Build history of the part. All positions in model axes, mm. Face numbers are marked on the shaded views. A direction names the side the tool comes from. Give positions to 0.01 mm unless a question says otherwise; leave off trailing zeros. Order: outer loops, then holes, each group sorted by start corner. A loop starts at its lowest first (then second) coordinate and runs counter-clockwise, first axis right, second up. Notation, with made-up numbers: (63, 68.5) - (71, 68.5) arc R30 cw to (71, 104.5) - close; hole circle Ø1 at (49, 87). An arc over 180 degrees is marked (long way). Use a Markdown table: item, result. Add a question column.
(1) Slice it at D-D (y = 1). Write the cut outline in (x, z), then the cut area to 3 significant figures.
(2) Flat gauge pins, fed straight in: pin 1 (5 mm diameter, centred on x = -2.5, z = -12.5, fed in from +Y); pin 2 (1.5 mm diameter, centred on y = 2.5, z = -15, fed in from +X); pin 3 (4.5 mm diameter, centred on x = 11, y = 2.5, fed in from -Z); pin 4 (1 mm diameter, centred on y = -1.5, z = 15.5, fed in from -X). Where does each tip first touch, or does it go through?
(3) Slice it at B-B (z = 12.5). Write the cut outline in (x, y).
(4) Mould opens along X. For the marked faces 1, 2, 3 and 4 say: +X half, -X half, draft (parallel to the pull), parting line (faces both ways), or undercut.
(5) Slice it at A-A (x = -2.5). Write the cut outline in (y, z), then the cut area to 3 significant figures.
(6) Slice it at C-C (y = -1.5). Write the cut outline in (x, z).
(7) Which spindle directions (+Z, -Z, +X, -X, +Y, -Y) get a long thin tool onto all of the face, cutting with end or side? Do the marked faces 5, 6, 7, 8 and 9. Say none if no direction does.
(8) Wall check: line 1 (Z direction, x = -2.5, y = 1.55); line 2 (Z direction, x = 11.25, y = 4); line 3 (X direction, y = -1.5, z = 16.5). Give the ranges that are in metal, low to high.
from build123d import *

# Parameters (mm, degrees)
EXTRUDE_1_DEPTH              = 10
SKETCH_2_W                   = 16
SKETCH_2_H                   = 6.92820323
EXTRUDE_2_DEPTH              = 10
SKETCH_3_W                   = 10
SKETCH_3_H                   = 6.92820323
CUT_EXTRUDE_1_DEPTH          = 1.5
CUT_EXTRUDE_2_DEPTH          = 1.92820323
EXTRUDE_3_DEPTH              = 10
SKETCH_6_W                   = 14.5
SKETCH_6_H                   = 5
EXTRUDE_4_DEPTH              = 10
HOLE_WIZARD_3_0_3_1_D        = 3
HOLE_WIZARD_3_0_3_1_DEPTH    = 10
HOLE_WIZARD_M5_1_D           = 5.5
HOLE_WIZARD_M5_1_DEPTH       = 9.237604307
HOLE_WIZARD_M5_1_CSINK_D     = 11.2
HOLE_WIZARD_M5_1_CSINK_ANGLE = 90
HOLE_WIZARD_3_0_3_2_D        = 3
HOLE_WIZARD_3_0_3_2_DEPTH    = 30
CHAMFER_1_SIZE               = 2


with BuildPart() as part:
    # 草图1 → 凸台-拉伸1 (new body)
    with BuildSketch(Plane.XY):
        Polygon((10, 5), (-10, 5), (-10, -1.92820323), (6, -1.92820323), (10, -4.237604307), (14, -1.92820323), (14, 2.690598923), align=None)
    extrude(amount=-EXTRUDE_1_DEPTH)

    # 草图2 → 凸台-拉伸2 (add)
    with BuildSketch(Plane.XY):
        with Locations((-2, 1.535898385)):
            Rectangle(SKETCH_2_W, SKETCH_2_H)
    extrude(amount=EXTRUDE_2_DEPTH)

    # 草图3 → 切除-拉伸1 (cut)
    with BuildSketch(Plane(origin=(6, 0, 0), x_dir=(0, 0, -1), z_dir=(1, 0, 0))):
        with Locations((-5, 1.535898385)):
            Rectangle(SKETCH_3_W, SKETCH_3_H)
    extrude(amount=-CUT_EXTRUDE_1_DEPTH, mode=Mode.SUBTRACT)

    # 草图4 → 切除-拉伸2 (cut)
    with BuildSketch(Plane.XZ.offset(1.92820323)):
        Polygon((4.5, 0), (4.5, 10), (-10, 10), (-10, -10), (6, -10), (6, 0), align=None)
    extrude(amount=-CUT_EXTRUDE_2_DEPTH, mode=Mode.SUBTRACT)

    # 草图5 → 凸台-拉伸3 (add)
    with BuildSketch(Plane.XY.offset(10)):
        Polygon((-10, 5), (10, 5), (14, 2.690598923), (14, -1.92820323), (10, -4.237604307), (6, -1.92820323), (6, 0), (-10, 0), align=None)
    extrude(amount=EXTRUDE_3_DEPTH)

    # 草图6 → 凸台-拉伸4 (add)
    with BuildSketch(Plane(origin=(0, 0, -10), x_dir=(-1, 0, 0), z_dir=(0, 0, -1))):
        with Locations((2.75, 2.5)):
            Rectangle(SKETCH_6_W, SKETCH_6_H)
    extrude(amount=EXTRUDE_4_DEPTH)

    # Ø3.0 (3) 直径孔1
    with Locations(Plane(origin=(0, 0, 10), x_dir=(-1, 0, 0), z_dir=(0, 0, -1))):
        with Locations((-10, 0.381197846)):
            Hole(HOLE_WIZARD_3_0_3_1_D / 2, depth=HOLE_WIZARD_3_0_3_1_DEPTH)

    # M5 平头机械螺钉的锥形沉头孔1
    with Locations(Plane(origin=(0, 5, 0), x_dir=(1, 0, 0), z_dir=(0, 1, 0))):
        with Locations((-2.5, 12.5), (-2.5, -12.5)):
            CounterSinkHole(HOLE_WIZARD_M5_1_D / 2, HOLE_WIZARD_M5_1_CSINK_D / 2, depth=HOLE_WIZARD_M5_1_DEPTH, counter_sink_angle=HOLE_WIZARD_M5_1_CSINK_ANGLE)

    # Ø3.0 (3) 直径孔2
    with Locations(Plane(origin=(0, 0, -10), x_dir=(-1, 0, 0), z_dir=(0, 0, -1))):
        with Locations((-10, 0.381197846)):
            Hole(HOLE_WIZARD_3_0_3_2_D / 2, depth=HOLE_WIZARD_3_0_3_2_DEPTH)

    # 倒角1
    # the kernel refuses this chamfer: 2 mm, written as the material it takes off along each edge
    with BuildSketch(Plane(origin=(-10, 5, -25.143365976), x_dir=(0.9996219169112968, 0.027495876610586487, 0), z_dir=(0, 0, 1))) as chamfer_1_piece_1:
        Polygon((CHAMFER_1_SIZE * 0.999621916911, -CHAMFER_1_SIZE * 0.0274958766106), (-CHAMFER_1_SIZE * 0.0274958766106, -CHAMFER_1_SIZE * 0.999621916911), (0, 0), align=None)
    extrude(amount=50.286731952, mode=Mode.SUBTRACT)


solid = part.part
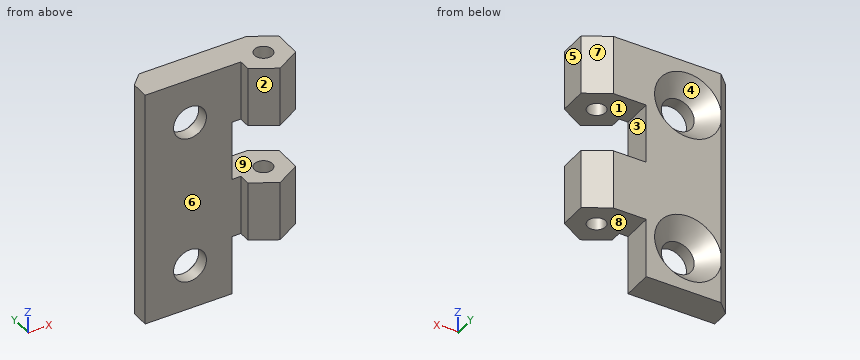
Solution:
| question | item | result |
|---|---|---|
| 1 | outline | (-10, -20) - (4.5, -20) - (4.5, -10) - (8.63, -10) - (8.63, 0) - (4.5, 0) - (4.5, 10) - (8.63, 10) - (8.63, 20) - (-10, 20) - close; (11.37, -10) - (14, -10) - (14, 0) - (11.37, 0) - close; (11.37, 10) - (14, 10) - (14, 20) - (11.37, 20) - close; hole circle Ø5.5 at (-2.5, -12.5); hole circle Ø5.5 at (-2.5, 12.5) |
| 1 | area | 668 mm2 |
| 2 | pin 1 | through |
| 2 | pin 2 | x = 4.5 |
| 2 | pin 3 | z = -10 |
| 2 | pin 4 | x = 6 |
| 3 | outline | (-10, 0) - (-5.25, 0) - (-5.25, 2.15) - (-8.05, 4.95) - (-10, 3) - close; (0.25, 0) - (6, 0) - (6, -1.93) - (10, -4.24) - (14, -1.93) - (14, 2.69) - (10, 5) - (3.1, 5) - (0.25, 2.15) - close; hole circle Ø3 at (10, 0.38) |
| 4 | face 1 | draft |
| 4 | face 2 | -X half |
| 4 | face 3 | +X half |
| 4 | face 4 | undercut |
| 5 | outline | (0, -20) - (5, -20) - (5, -18.1) - (2.15, -15.25) - (0, -15.25) - close; (0, -9.75) - (2.15, -9.75) - (5, -6.9) - (5, 6.9) - (2.15, 9.75) - (0, 9.75) - close; (0, 15.25) - (2.15, 15.25) - (5, 18.1) - (5, 20) - (0, 20) - close |
| 5 | area | 129 mm2 |
| 6 | outline | (6, -10) - (14, -10) - (14, 0) - (6, 0) - close; (6, 10) - (14, 10) - (14, 20) - (6, 20) - close |
| 7 | face 5 | +Z, -Z, +X, +Y, -Y |
| 7 | face 6 | +Z, -Z, -X, -Y |
| 7 | face 7 | +Z, -Z, +X, +Y |
| 7 | face 8 | -Z, +X, +Y, -Y |
| 7 | face 9 | +X, +Y, -Y |
| 8 | line 1 | -20 to -15.25, -9.75 to 9.75, 15.25 to 20 |
| 8 | line 2 | -10 to 0, 10 to 20 |
| 8 | line 3 | 6 to 14 |
